```python
from build123d import *

# Parameters (mm, degrees)
SKETCH1_W = 60
SKETCH1_H = 15


with BuildPart() as part:
    # Эскиз1 → Revolve 449 (revolve)
    with BuildSketch(Plane.XY, mode=Mode.PRIVATE) as revolve_449_sk:
        with BuildLine():
            Line((5, 76.341055046), (60, 76.341055046))
            Line((60, 76.341055046), (60, 66.341055046))
            Line((60, 66.341055046), (15, 66.341055046))
            ThreePointArc((15, 66.341055046), (11.464466094, 64.876588952), (10, 61.341055046))
            Line((10, 61.341055046), (10, 56.341055046))
            Line((10, 56.341055046), (0, 56.341055046))
            Line((0, 56.341055046), (0, 71.341055046))
            Line((0, 71.341055046), (5, 71.341055046))
            Line((5, 71.341055046), (5, 76.341055046))
        make_face()
    revolve(revolve_449_sk.sketch.rotate(Axis((-60, 97.731625762, 0), (0, -1, 0)), 180), axis=Axis((-60, 97.731625762, 0), (0, -1, 0)))

    # Sketch1 → Revolve1 (revolve)
    with BuildSketch(Plane.XY):
        with Locations((-30, 63.841055046)):
            Rectangle(SKETCH1_W, SKETCH1_H)
    revolve(axis=Axis((-60, 66.341055046, 0), (0, 1, 0)))


solid = part.part
```
Input: part model. Units: mm. Frame: model coordinates. A direction names the side the tool comes from. Give positions to 0.01 mm unless a question says otherwise; leave off trailing zeros. Loops run counter-clockwise (first coordinate to the right, second up) from the corner with the lowest first, then second, coordinate; pieces in that order, holes last.
1) Contact query for flat-ended pins moving along their axis: pin 1 (12 mm diameter, centred on x = -80, z = -53.5, fed in from +Y); pin 2 (6 mm diameter, centred on x = -26.5, y = 61, fed in from +Z); pin 3 (5 mm diameter, centred on y = 69.5, z = 70.5, fed in from -X). Output: stop coordinate, or through.
A:
pin 1: stops at y = 71.34
pin 2: stops at z = 63.01
pin 3: stops at x = -158.87
2) Mould query, pull axis X, two halves, no side actions, for faces 4 (the cylindrical face through (-44.825, 58.806, 68.335)), 5 (the cylindrical face through (-122, 73.88, -19.52)), 6 (the flat face through (-8, 76.341, 52)). Classes: released by +X, released by -X, zero draft, split by the parting line, or undercut.
A:
face 4: split by the parting line
face 5: undercut
face 6: zero draft
3) Line query: L1, parallel to Z at x = -60, y = 75.3; L2, parallel to Y at x = 12, z = 56; L3, parallel to Y at x = -77, z = 2. Output: solid intervals per line, ascending.
A:
L1: z = -120 to -65, 65 to 120
L2: y = 66.34 to 76.34
L3: y = 56.34 to 71.34
4) Section query A-A on z = 0. Return the cut outline in (x, y).
A:
outline: (-180, 66.34) - (-135, 66.34) arc R5 cw to (-130, 61.34) - (-130, 56.34) - (10, 56.34) - (10, 61.34) arc R5 cw to (15, 66.34) - (60, 66.34) - (60, 76.34) - (5, 76.34) - (5, 71.34) - (-125, 71.34) - (-125, 76.34) - (-180, 76.34) - close
5) Section query B-B on x = -60. Return the cut outline in (y, z), and give its area (3 significant figures).
A:
outline: (56.34, -70) - (61.34, -70) arc R5 cw to (66.34, -75) - (66.34, -120) - (76.34, -120) - (76.34, -65) - (71.34, -65) - (71.34, 65) - (76.34, 65) - (76.34, 120) - (66.34, 120) - (66.34, 75) arc R5 cw to (61.34, 70) - (56.34, 70) - close
area: 3,160 mm2
6) Section query D-D on z = -87. Return the cut outline in (x, y).
A:
outline: (-142.65, 66.34) - (22.65, 66.34) - (22.65, 76.34) - (-142.65, 76.34) - close
7) Reachability of faces 1 (the flat face through (-5, 66.341, 52)), 2 (the cylindrical face through (-170.85, 71.27, 45.96)), 3 (the flat face through (-61, 71.341, -1)) from +Z, -Z, +X, -X, +Y, -Y: full face, straight path, thin tool, end or side. Return the list, or none.
A:
face 1: -Y
face 2: +Y, -Y
face 3: +Y
8) Section query C-C on x = -142. Return the cut outline in (y, z), and give its area (3 significant figures).
A:
outline: (66.34, -87.61) - (76.34, -87.61) - (76.34, 87.61) - (66.34, 87.61) - close
area: 1,750 mm2
